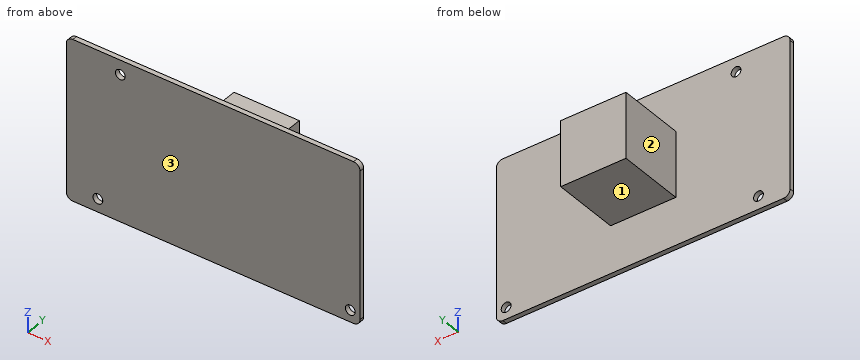
from build123d import *

# Parameters (mm, degrees)
SKETCH1_W             = 90
SKETCH1_H             = 49
BOSS_EXTRUDE1_DEPTH   = 1.5
FILLET1_R             = 2
F_1_0MM_DOWEL_HOLE1_D = 3
SKETCH4_W             = 20
SKETCH4_H             = 20
BOSS_EXTRUDE2_DEPTH   = 22


with BuildPart() as part:
    # Sketch1 → Boss-Extrude1 (new body)
    with BuildSketch(Plane(origin=(0, 0, 0), x_dir=(1, 0, 0), z_dir=(0, 1, 0))):
        Rectangle(SKETCH1_W, SKETCH1_H)
    extrude(amount=BOSS_EXTRUDE1_DEPTH)

    # Fillet1
    fillet1_edges = [part.edges().sort_by_distance(p)[0] for p in [
        (45, 0.75, 24.5),
        (-45, 0.75, 24.5),
        (-45, 0.75, -24.5),
        (45, 0.75, -24.5),
    ]]
    fillet(fillet1_edges, radius=FILLET1_R)

    # Ø1.0mm Dowel Hole1 (through all)
    with Locations(Plane(origin=(0, 1.5, 0), x_dir=(1, 0, 0), z_dir=(0, 1, 0))):
        with Locations((-35.325, 20.5), (42, 20.9), (-28.45, -20.1)):
            Hole(F_1_0MM_DOWEL_HOLE1_D / 2)

    # Sketch4 → Boss-Extrude2 (add)
    with BuildSketch(Plane.XZ):
        Rectangle(SKETCH4_W, SKETCH4_H)
    extrude(amount=-BOSS_EXTRUDE2_DEPTH)


solid = part.part
For this review, take the finished solid that the model builds, in its own axes (mm). Face numbers are marked on the shaded views. A direction names the side the tool comes from. Give positions to 0.01 mm unless a question says otherwise; leave off trailing zeros. Order: outer loops, then holes, each group sorted by start corner. A loop starts at its lowest first (then second) coordinate and runs counter-clockwise, first axis right, second up. Notation, with made-up numbers: (84, 22.5) - (139, 22.5) arc R15 ccw to (139, 40.5) - close; hole circle Ø10 at (83.25, 52.5). An arc over 180 degrees is marked (long way). Answer as a JSON object with one key per item and string values. Group by question number.
Item 1: Clearance check with flat-ended pins moving along their axes: pin 1 Ø3.5 at (x, z) = (42, -20.9) entering from -Y; pin 2 Ø2.5 at (x, z) = (-35.325, -20.5) entering from -Y; pin 3 Ø6 at (x, y) = (4.5, 12) entering from +Z; pin 4 Ø4 at (x, z) = (-28.45, 20.1) entering from +Y. State where each tip first meets the part, or that it passes through.
Item 2: Wall thickness on line 1 along X through (y, z) = (0.85, -20.9); line 2 along X through (y, z) = (1, -20.5) (3 decimals); line 3 along X through (y, z) = (5.5, -0.5): over which ranges is each line inside the solid? List them lowest first.
Item 3: Take a section at C-C on x = 7.5. Give the boundary of the cut face in (y, z).
Item 4: Take a section at D-D on z = -1.5. Give the boundary of the cut face in (x, y).
Item 5: Machinability: for the marked faces 1, 2 and 3, which of the approach directions +Z, -Z, +X, -X, +Y, -Y give a long, thin tool a straight path to every point of the face, cutting with its end or side? Answer none if there is none.
Item 6: Take a section at B-B on x = 42. Give the boundary of the cut face in (y, z), and give its area (3 significant figures).
Item 7: Take a section at A-A on z = 20.1. Give the boundary of the cut face in (x, y).
Reported:
{
 "1": {"pin 1": "y = 0", "pin 2": "through", "pin 3": "z = 10", "pin 4": "y = 1.5"},
 "2": {"line 1": "-45 to -36.77, -33.88 to 40.5, 43.5 to 45", "line 2": "-45 to -36.825, -33.825 to 40.554, 43.446 to 45", "line 3": "-10 to 10"},
 "3": {"outline": "(0, -24.5) - (1.5, -24.5) - (1.5, -10) - (22, -10) - (22, 10) - (1.5, 10) - (1.5, 24.5) - (0, 24.5) - close"},
 "4": {"outline": "(-45, 0) - (45, 0) - (45, 1.5) - (10, 1.5) - (10, 22) - (-10, 22) - (-10, 1.5) - (-45, 1.5) - close"},
 "5": {"face 1": "-Z, +X, -X, +Y", "face 2": "+Z, -Z, -X, +Y", "face 3": "+Z, -Z, +X, -X, -Y"},
 "6": {"outline": "(0, -24.5) - (1.5, -24.5) - (1.5, -22.4) - (0, -22.4) - close; (0, -19.4) - (1.5, -19.4) - (1.5, 24.5) - (0, 24.5) - close", "area": "69.0 mm^2"},
 "7": {"outline": "(-45, 0) - (-29.95, 0) - (-29.95, 1.5) - (-45, 1.5) - close; (-26.95, 0) - (45, 0) - (45, 1.5) - (-26.95, 1.5) - close"}
}
